Work out the finished part from the listing and answer in its coordinate system (mm). A direction names the side the tool comes from. Coordinates: 2 decimals unless noted, no trailing zeros. Write each loop counter-clockwise with the first axis right and the second up, starting at its lowest first coordinate (ties: lowest second). Pieces come first, ordered by that corner, then holes. Notation, with made-up numbers: (-0.75, -3.75) - (49.25, -3.75) arc R19 cw to (49.25, 8.25) - close; hole circle Ø2 at (-38, 84). An arc over 180 degrees is marked (long way). Use a Markdown table: item, result. Add a question column.
(1) The part is cut by section A-A, the plane x = 0. Give the vertices of the cut face in (y, z), then the cut area to 3 significant figures.
(2) For a pull along Z with two mould halves and no side action, classify faces 5 (the face through (-9.283, 20, -16)), 6 (the face through (-45, 120, -19)), 7 (the face through (1.099, 59.16, -49.988)) as released by +Z, released by -Z, zero draft, split by the parting line, or undercut.
(3) The part is cut by section C-C, the plane z = 33. Give the vertices of the cut face in (x, y), then the cut area to 3 significant figures.
(4) The part is cut by section B-B, the plane y = 62. Give the vertices of the cut face in (x, z).
(5) A tool of negligible diameter and unlimited length cuts with its end or side. For faces 1 (the face through (-1.38, 97.8, 49.16)), 2 (the face through (-12, 25, -22.3)), 3 (the face through (-12.2, 25, -19)), 4 (the face through (-1, 0, 10)), from which of +Z, -Z, +X, -X, +Y, -Y can it reach the whole face along a straight path? Write none if from no direction.
(6) The part is cut by section D-D, the plane y = 104. Give the vertices of the cut face in (x, z).
(7) Given pin 1 Ø10 at (x, z) = (-39.5, 16.5) entering from +Y; pin 2 Ø1.6 at (y, z) = (0.5, -27.5) entering from -X; pin 3 Ø1.5 at (x, z) = (8, -11.5) entering from -Y; pin 4 Ø5 at (y, z) = (107, -30) entering from +X, each flat-ended and moving along its own axis, determine where each tip first touches the part or whether it passes through.
(8) Find the intervals of material crossed by line 1 (Y direction, x = 0, z = 49); line 2 (Z direction, x = -9.5, y = 26.5); line 3 (X direction, y = 106.5, z = 4.5), in increasing order. Write a range as from..to.
from build123d import *

# Parameters (mm, degrees)
BOSS_EXTRUDE1_DEPTH = 120
CUT_EXTRUDE1_DEPTH  = 118
SKETCH18_R          = 6.35
CUT_EXTRUDE9_DEPTH  = 8
CUT_EXTRUDE10_START = -2
CUT_EXTRUDE10_DEPTH = 2
BOSS_EXTRUDE2_DEPTH = 48
CHAMFER1_SIZE       = 2
CHAMFER1_SIZE2      = 7.464101615
SKETCH20_W          = 5.5
SKETCH20_H          = 29.700000001
SKETCH20_W_2        = 8
SKETCH20_H_2        = 3
CUT_EXTRUDE11_DEPTH = 165.012194669


# Read off the part's stored shape, not the designer's step: Cut-Extrude10, Boss-Extrude2
with BuildPart() as part:
    # Sketch2 → Boss-Extrude1 (new body)
    with BuildSketch(Plane(origin=(0, 0, 0), x_dir=(1, 0, 0), z_dir=(0, 1, 0))):
        with BuildLine():
            Line((-50, 0), (-50, -50))
            Line((-50, -50), (50, -50))
            Line((50, -50), (50, 0))
            ThreePointArc((50, 0), (0, 50), (-50, 0))
        make_face()
    extrude(amount=BOSS_EXTRUDE1_DEPTH)

    # Sketch3 → Cut-Extrude1 (cut)
    with BuildSketch(Plane(origin=(0, 120, 0), x_dir=(1, 0, 0), z_dir=(0, 1, 0))):
        with BuildLine():
            Line((-48.3, 0), (-48.3, -48.3))
            Line((-48.3, -48.3), (48.3, -48.3))
            Line((48.3, -48.3), (48.3, 0))
            ThreePointArc((48.3, 0), (0, 48.3), (-48.3, 0))
        make_face()
    extrude(amount=-CUT_EXTRUDE1_DEPTH, mode=Mode.SUBTRACT)

    # Sketch18 → Cut-Extrude9 (cut)
    with BuildSketch(Plane.XY.offset(50)):
        with Locations((0, 104)):
            Circle(SKETCH18_R)
    extrude(amount=-CUT_EXTRUDE9_DEPTH, mode=Mode.SUBTRACT)

    # Cut-Extrude10 outline → Cut-Extrude10 (cut)
    with BuildSketch(Plane(origin=(0, 2, 0), x_dir=(1, 0, 0), z_dir=(0, 1, 0)).offset(CUT_EXTRUDE10_START)):
        Polygon((12.2, 16.55), (12.2, 21.3), (9.282585541, 21.3), (9.282585541, 22.3), (11.241292771, 22.3), (11.241292771, 29.388121527), (13.2, 29.388121527), (13.2, 40.3), (-13.2, 40.3), (-13.2, 29.388121527), (-11.241292771, 29.388121527), (-11.241292771, 22.3), (-9.282585541, 22.3), (-9.282585541, 21.3), (-12.2, 21.3), (-12.2, 16.55), align=None)
    extrude(amount=CUT_EXTRUDE10_DEPTH, mode=Mode.SUBTRACT)

    # Boss-Extrude2 outline → Boss-Extrude2 (add)
    with BuildSketch(Plane(origin=(0, 2, 0), x_dir=(1, 0, 0), z_dir=(0, 1, 0))):
        Polygon((9.282585541, 21.3), (12.2, 21.3), (12.2, 16.55), (9.282585541, 16.55), (9.282585541, 15.55), (13.2, 15.55), (13.2, 22.3), (9.282585541, 22.3), align=None)
        Polygon((-9.282585541, 15.55), (-9.282585541, 16.55), (-12.2, 16.55), (-12.2, 21.3), (-9.282585541, 21.3), (-9.282585541, 22.3), (-13.2, 22.3), (-13.2, 15.55), align=None)
    extrude(amount=BOSS_EXTRUDE2_DEPTH)

    # Chamfer1
    chamfer1_edges = [part.edges().sort_by_distance(p)[0] for p in [
        (13.2, 2, -18.925),
        (11.24129277, 2, -15.55),
        (-13.2, 2, -18.925),
        (-11.24129277, 2, -15.55),
    ]]
    chamfer1_side = [part.faces().sort_by_distance(p)[0] for p in [
        (0, 2, 7.094220812),
    ]]
    chamfer(chamfer1_edges, length=CHAMFER1_SIZE, length2=CHAMFER1_SIZE2, reference=chamfer1_side[0])

    # Sketch20 → Cut-Extrude11 (cut, through all)
    with BuildSketch(Plane(origin=(50, 0, 0), x_dir=(0, 0, -1), z_dir=(1, 0, 0))):
        with Locations((3.25, 67.984146729)):
            Rectangle(SKETCH20_W, SKETCH20_H)
        with Locations((0, 111.353074805)):
            Rectangle(SKETCH20_W_2, SKETCH20_H_2)
    extrude(amount=-CUT_EXTRUDE11_DEPTH, mode=Mode.SUBTRACT)


solid = part.part
Model answer:
| question | item | result |
|---|---|---|
| 1 | outline | (0, -50) - (120, -50) - (120, -48.3) - (2, -48.3) - (2, -40.3) - (0, -40.3) - close; (0, -16.55) - (2, -16.55) - (2, 48.3) - (97.65, 48.3) - (97.65, 50) - (0, 50) - close; (110.35, 48.3) - (120, 48.3) - (120, 50) - (110.35, 50) - close |
| 1 | area | 532 mm^2 |
| 2 | face 5 | undercut |
| 2 | face 6 | zero draft |
| 2 | face 7 | released by -Z |
| 3 | outline | (-50, 0) - (50, 0) - (50, 120) - (48.3, 120) - (48.3, 2) - (-48.3, 2) - (-48.3, 120) - (-50, 120) - close |
| 3 | area | 601 mm^2 |
| 4 | outline | (-50, -0.5) - (-48.3, -0.5) arc R48.3 cw to (-48.3, 0) - (-48.3, 48.3) - (48.3, 48.3) - (48.3, 0) arc R48.3 cw to (48.3, -0.5) - (50, -0.5) arc R50 ccw to (50, 0) - (50, 50) - (-50, 50) - (-50, 0) arc R50 ccw to start; (-49.64, -6) arc R50 ccw to (49.64, -6) - (47.93, -6) arc R48.3 cw to (-47.93, -6) - close |
| 5 | face 1 | +Z |
| 5 | face 2 | +Y |
| 5 | face 3 | +Y, -Y |
| 5 | face 4 | +Z, -Z, +X, -X, -Y |
| 6 | outline | (-50, 0) arc R50 ccw to (50, 0) - (50, 50) - (6.35, 50) - (6.35, 48.3) - (48.3, 48.3) - (48.3, 0) arc R48.3 cw to (-48.3, 0) - (-48.3, 48.3) - (-6.35, 48.3) - (-6.35, 50) - (-50, 50) - close |
| 7 | pin 1 | y = 2 |
| 7 | pin 2 | x = -42.27 |
| 7 | pin 3 | y = 0 |
| 7 | pin 4 | x = 41.76 |
| 8 | line 1 | 0..97.65, 110.35..120 |
| 8 | line 2 | -49.09..-47.36, -22.3..-21.3, -16.55..-15.55, 48.3..50 |
| 8 | line 3 | -50..-48.3, 48.3..50 |
